Geometry: final body of the model. Coordinates: model frame, mm. Face numbers are marked on the shaded views. A direction names the side the tool comes from. Give positions to 0.01 mm unless a question says otherwise; leave off trailing zeros. Write each loop counter-clockwise with the first axis right and the second up, starting at its lowest first coordinate (ties: lowest second). Pieces come first, ordered by that corner, then holes. Notation, with made-up numbers: (-19, 62) -> (34, 62) arc R5 cw to (34, 71) -> close; hole circle Ø8 at (-19, 49). An arc over 180 degrees is marked (long way). Answer as a JSON object with one key per item and string values.
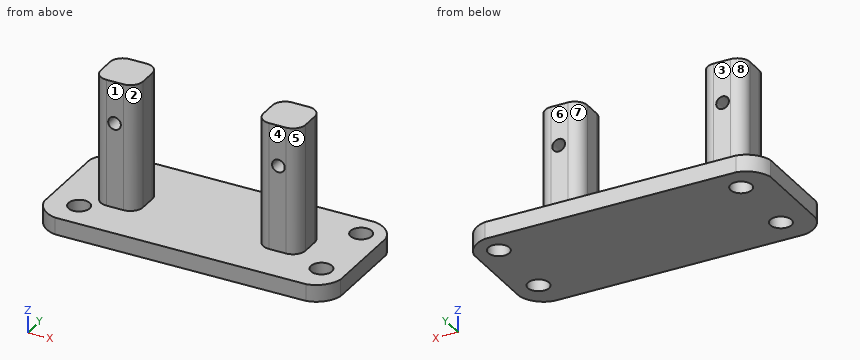
from build123d import *

# Parameters (mm, degrees)
SKETCH_W        = 70
SKETCH_H        = 30
PAD_DEPTH       = 4
PAD001_DEPTH    = 30
SKETCH003_R     = 1.5
POCKET_DEPTH    = 10
SKETCH004_R     = 2.5
HOLE_DEPTH      = 25
POCKET001_DEPTH = 5


with BuildPart() as part:
    # Sketch → Pad (new body)
    with BuildSketch(Plane.XY):
        Rectangle(SKETCH_W, SKETCH_H)
    extrude(amount=PAD_DEPTH)

    # Sketch001 → Pad001 (join)
    with BuildSketch(Plane.XY.offset(4)):
        with BuildLine():
            Line((-25.674894, 1.559909), (-25.674894, -2.440091))
            ThreePointArc((-25.674894, -2.440091), (-24.796214, -4.561411), (-22.674894, -5.440091))
            Line((-22.674894, -5.440091), (-18.674894, -5.440091))
            ThreePointArc((-18.674894, -5.440091), (-16.553574, -4.561411), (-15.674894, -2.440091))
            Line((-15.674894, -2.440091), (-15.674894, 1.559909))
            ThreePointArc((-15.674894, 1.559909), (-16.553574, 3.681229), (-18.674894, 4.559909))
            Line((-18.674894, 4.559909), (-22.674894, 4.559909))
            ThreePointArc((-22.674894, 4.559909), (-24.796214, 3.681229), (-25.674894, 1.559909))
        make_face()
        with BuildLine():
            Line((12.775577, 1.472262), (12.775577, -2.527736))
            ThreePointArc((12.775577, -2.527736), (13.654257, -4.649056), (15.775577, -5.527736))
            Line((15.775577, -5.527736), (19.775106, -5.527736))
            ThreePointArc((19.775106, -5.527736), (21.896426, -4.649056), (22.775106, -2.527736))
            Line((22.775106, -2.527736), (22.775106, 1.472262))
            ThreePointArc((22.775106, 1.472262), (21.896426, 3.593582), (19.775106, 4.472262))
            Line((19.775106, 4.472262), (15.775577, 4.472262))
            ThreePointArc((15.775577, 4.472262), (13.654257, 3.593582), (12.775577, 1.472262))
        make_face()
    extrude(amount=PAD001_DEPTH)

    # Sketch003 → Pocket (cut, symmetric)
    with BuildSketch(Plane.XZ.offset(3.853326)):
        with Locations((-20.799536, 24.110664)):
            Circle(SKETCH003_R)
        with Locations((17.973553, 24.375628)):
            Circle(SKETCH003_R)
    extrude(amount=POCKET_DEPTH, both=True, mode=Mode.SUBTRACT)

    # Sketch004 (on Face5 of Pocket) → Hole (cut)
    with BuildSketch(Plane.XY.offset(4)):
        with Locations((29.484156, 9.351145)):
            Circle(SKETCH004_R)
        with Locations((29.302721, -7.648855)):
            Circle(SKETCH004_R)
        with Locations((-27.515844, 8.851251)):
            Circle(SKETCH004_R)
        with Locations((-27.697279, -8.148749)):
            Circle(SKETCH004_R)
    extrude(amount=-HOLE_DEPTH, mode=Mode.SUBTRACT)

    # Sketch005 (on Face5 of Hole) → Pocket001 (cut)
    with BuildSketch(Plane.XY.offset(4)):
        with BuildLine():
            ThreePointArc((-29.5254, 15.019082), (-33.217927, 13.152465), (-35.081265, 9.458282))
            Line((-35.081265, 9.458282), (-35.081265, 15.019082))
            Line((-35.081265, 15.019082), (-29.5254, 15.019082))
        make_face()
        with BuildLine():
            ThreePointArc((35.081265, 9.458282), (33.217927, 13.152465), (29.5254, 15.019082))
            Line((35.081265, 15.019082), (29.5254, 15.019082))
            Line((35.081265, 9.458282), (35.081265, 15.019082))
        make_face()
        with BuildLine():
            ThreePointArc((-35.081265, -9.458282), (-33.217927, -13.152465), (-29.5254, -15.019082))
            Line((-35.081265, -15.019082), (-29.5254, -15.019082))
            Line((-35.081265, -9.458282), (-35.081265, -15.019082))
        make_face()
        with BuildLine():
            ThreePointArc((29.5254, -15.019082), (33.217927, -13.152465), (35.081265, -9.458282))
            Line((35.081265, -9.458282), (35.081265, -15.019082))
            Line((35.081265, -15.019082), (29.5254, -15.019082))
        make_face()
    extrude(amount=-POCKET001_DEPTH, mode=Mode.SUBTRACT)


solid = part.part
Q1. Material intervals for L1, parallel to Z at x = -5, y = 11; L2, parallel to Y at x = -18.5, z = 13; L3, parallel to X at y = 3, z = 15, sorted ascending. Write a range as from..to.
Values:
{"L1": "0..4", "L2": "-5.43..4.55", "L3": "-25.31..-16.04, 13.19..22.36"}
Q2. First-contact query: P1, Ø3, axis at x = 12.5, y = 10.5, coming from the +Z side; P2, Ø3, axis at x = 17.5, z = 23, coming from the -Y side; P3, Ø10, axis at y = -6, z = 16, coming from the -X side. Flat tips, straight axial feed; report the tip coordinate or a pass-through.
Values:
{"P1": "z = 4", "P2": "y = -5.53", "P3": "x = -25.67"}
Q3. Cut plane C-C (z = 2.5). Return the cut outline in (x, y), and give its area (3 significant figures).
Values:
{"outline": "(-35, -9.9) arc R6.62 ccw to (-29.64, -15) -> (29.64, -15) arc R6.62 ccw to (35, -9.9) -> (35, 9.9) arc R6.62 ccw to (29.64, 15) -> (-29.64, 15) arc R6.62 ccw to (-35, 9.9) -> close; hole circle Ø5 at (-27.7, -8.15); hole circle Ø5 at (-27.52, 8.85); hole circle Ø5 at (29.3, -7.65); hole circle Ø5 at (29.48, 9.35)", "area": "1,990 mm²"}
Q4. Cut plane B-B (y = -1). Return the cut outline in (x, z), and give its area (3 significant figures).
Values:
{"outline": "(-35, 0) -> (35, 0) -> (35, 4) -> (22.78, 4) -> (22.78, 34) -> (12.78, 34) -> (12.78, 4) -> (-15.67, 4) -> (-15.67, 34) -> (-25.67, 34) -> (-25.67, 4) -> (-35, 4) -> close; hole circle Ø3 at (-20.8, 24.11); hole circle Ø3 at (17.97, 24.38)", "area": "866 mm²"}
Q5. Set-up query: the marked faces 1, 2, 3, 4 and 5. Return all of +Z, -Z, +X, -X, +Y, -Y with unobstructed straight access to the full face (end or side cutting, diameter ignored); none if empty.
Values:
{"face 1": "+Z, -X, -Y", "face 2": "+Z, -Y", "face 3": "+Z, +X, -X, +Y", "face 4": "+Z, +X, -X, -Y", "face 5": "+Z, +X, -Y"}
Q6. Cut plane D-D (x = 5.5). Return the cut outline in (y, z).
Values:
{"outline": "(-15, 0) -> (15, 0) -> (15, 4) -> (-15, 4) -> close"}
Q7. Mould query, pull axis X, two halves, no side actions, for the marked faces 6, 7 and 8. Classes: pulls with the +X half, pulls with the -X half, needs draft (parallel to the pull), parting line crosses it, or undercut.
Values:
{"face 6": "needs draft", "face 7": "undercut", "face 8": "pulls with the -X half"}
Q8. Cut plane A-A (z = 13). Return the cut outline in (x, y), and give its area (3 significant figures).
Values:
{"outline": "(-25.67, -2.44) arc R3 ccw to (-22.67, -5.44) -> (-18.67, -5.44) arc R3 ccw to (-15.67, -2.44) -> (-15.67, 1.56) arc R3 ccw to (-18.67, 4.56) -> (-22.67, 4.56) arc R3 ccw to (-25.67, 1.56) -> close; (12.78, -2.53) arc R3 ccw to (15.78, -5.53) -> (19.78, -5.53) arc R3 ccw to (22.78, -2.53) -> (22.78, 1.47) arc R3 ccw to (19.78, 4.47) -> (15.78, 4.47) arc R3 ccw to (12.78, 1.47) -> close", "area": "185 mm²"}
